```python
from build123d import *

# Parameters (mm, degrees)
BOSS_EXTRUDE1_START = 48
BOSS_EXTRUDE1_DEPTH = 10


with BuildPart() as part:
    # Sketch1 → Boss-Extrude1 (new body)
    with BuildSketch(Plane.XY.offset(BOSS_EXTRUDE1_START)):
        Polygon((-35.751247902, 1576.485487398), (-35.751247902, 1705.542913165), (56.982876999, 1705.542913165), (56.982876999, 1576.485487398), (216.535268781, 1576.485487398), (216.535268781, 1788.738422577), (-215.875298803, 1788.738422577), (-215.875298803, 1576.485487398), align=None)
    extrude(amount=BOSS_EXTRUDE1_DEPTH)


solid = part.part
```
Could you check a few things on this model? Use its own coordinates, in mm. A direction names the side the tool comes from. Round coordinates to 2 decimals unless told otherwise and drop trailing zeros. Order: outer loops, then holes, each group sorted by start corner. A loop starts at its lowest first (then second) coordinate and runs counter-clockwise, first axis right, second up. Notation, with made-up numbers: M 1,62.5 L 47,62.5 A21 ccw 47,70.5 Z; hole C -35,12 d11. An arc over 180 degrees is marked long. One line per question, with ' | ' between items. Start each with the question number.
(1) Suppose I cut it at A-A on y = 1597.5. List the corners of the cut face in (x, z) for me, then the cut area to 3 significant figures.
(2) Suppose I cut it at B-B on z = 49.5. List the corners of the cut face in (x, y) for me, then the cut area to 3 significant figures.
(3) Please list where these lines run through material, in increasing order: line 1 along X through (y, z) = (1611.5, 54.5); line 2 along Y through (x, z) = (-18.5, 52.25).
(4) For faces 1 (the face through (-3, 1708, 48)), 2 (the face through (10, 1705.543, 53)), which set-ups out of +Z, -Z, +X, -X, +Y, -Y let a thin tool reach every point of the face, with its end or its side?
(5) Suppose I cut it at C-C on x = 2.5. List the corners of the cut face in (y, z) for me.
Geometry results:
1) outline: M -215.88,48 L -35.75,48 L -35.75,58 L -215.88,58 Z; M 56.98,48 L 216.54,48 L 216.54,58 L 56.98,58 Z | area: 3,400 mm²
2) outline: M -215.88,1576.49 L -35.75,1576.49 L -35.75,1705.54 L 56.98,1705.54 L 56.98,1576.49 L 216.54,1576.49 L 216.54,1788.74 L -215.88,1788.74 Z | area: 79,800 mm²
3) line 1: -215.88 to -35.75, 56.98 to 216.54 | line 2: 1705.54 to 1788.74
4) face 1: -Z, +X, -X, +Y, -Y | face 2: +Z, -Z, -Y
5) outline: M 1705.54,48 L 1788.74,48 L 1788.74,58 L 1705.54,58 Z
